The drawing under review shows one solid part. Ordinate dimensions are in mm from its lowest x, y, z. Give positions to 0.01 mm unless a question says otherwise; leave off trailing zeros. Write each loop counter-clockwise with the first axis right and the second up, starting at its lowest first coordinate (ties: lowest second). Pieces come first, ordered by that corner, then holes. Notation, with made-up numbers: (30.5, 85.5) -> (81.5, 85.5) arc R18 ccw to (81.5, 120.5) -> close; hole circle Ø9 at (-35, -11.5). An arc over 180 degrees is marked (long way). Use CSV: the item, a comma, the result in double quotes.
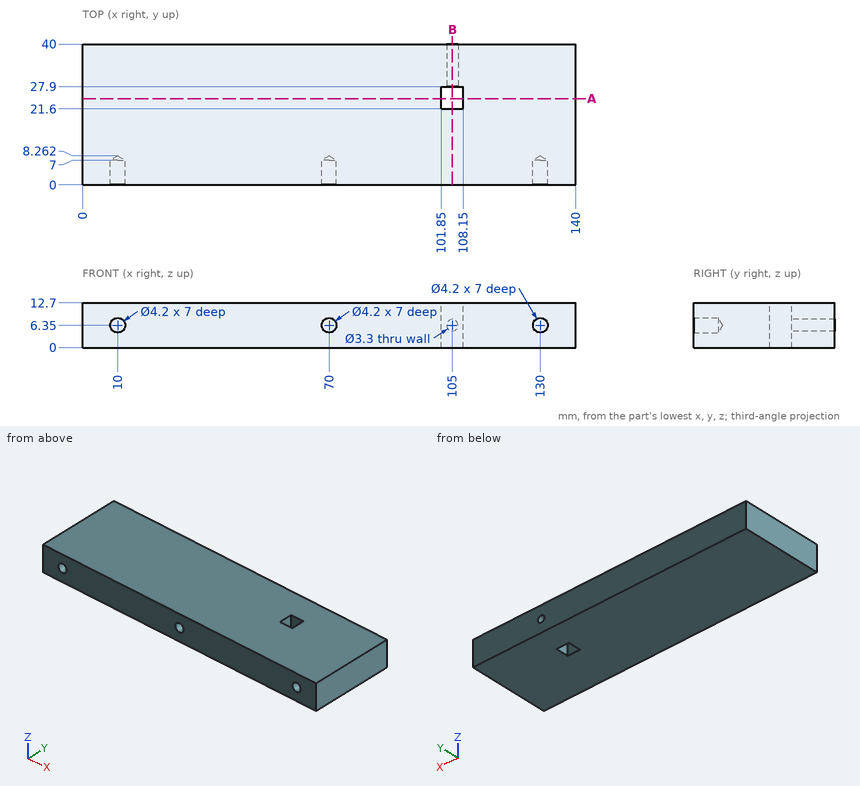
(1) Clearance check with a flat-ended pin moving along its axis: pin 1 (3.5 mm diameter, centred on x = 70, z = 6.35, fed in from -Y). State where the tip first meets the part, or that it passes through.
Established:
pin 1,"stops at y = 7.21"
(2) Take a section at A-A (y = 24.5). Write out the cut boundary in (x, z).
Established:
outline,"(0, 0) -> (101.85, 0) -> (101.85, 12.7) -> (0, 12.7) -> close; (108.15, 0) -> (140, 0) -> (140, 12.7) -> (108.15, 12.7) -> close"
(3) For line 1 along X through (y, z) = (2.75, 6.35); line 2 along Z through (x, y) = (105, 37.5); line 3 along X through (y, z) = (35, 6.35), list the stretches that pass through material, from the lowest coordinate up. Write a range as [from, to].
Established:
line 1,"x = [0, 7.9], [12.1, 67.9], [72.1, 127.9], [132.1, 140]"
line 2,"z = [0, 4.7], [8, 12.7]"
line 3,"x = [0, 103.35], [106.65, 140]"
(4) Take a section at B-B (x = 105). Write out the cut boundary in (y, z).
Established:
outline,"(0, 0) -> (21.6, 0) -> (21.6, 12.7) -> (0, 12.7) -> close; (27.9, 0) -> (40, 0) -> (40, 4.7) -> (27.9, 4.7) -> close; (27.9, 8) -> (40, 8) -> (40, 12.7) -> (27.9, 12.7) -> close"
